Here's how the part is built. I have some questions about the finished solid (model axes, mm). Give positions to 0.01 mm unless a question says otherwise; leave off trailing zeros. Order: outer loops, then holes, each group sorted by start corner. A loop starts at its lowest first (then second) coordinate and runs counter-clockwise, first axis right, second up.
from build123d import *

# Parameters (mm, degrees)
SKETCH1_W           = 73
SKETCH1_H           = 30
SKETCH1_W_2         = 7
SKETCH1_H_2         = 2
SKETCH1_W_3         = 2
SKETCH1_H_3         = 7
BOSS_EXTRUDE1_DEPTH = 2
CUT_EXTRUDE1_DEPTH  = 10
SKETCH6_R           = 2
CUT_EXTRUDE2_DEPTH  = 19


with BuildPart() as part:
    # Sketch1 → Boss-Extrude1 (new body)
    with BuildSketch(Plane(origin=(0, 0, 0), x_dir=(1, 0, 0), z_dir=(0, 1, 0))):
        with Locations((-11.269774173, -9.91409445)):
            Rectangle(SKETCH1_W, SKETCH1_H)
        with Locations((-39.269774173, -16.41409445)):
            Rectangle(SKETCH1_W_2, SKETCH1_H_2, mode=Mode.SUBTRACT)
        with Locations((-39.269774173, -3.41409445)):
            Rectangle(SKETCH1_W_2, SKETCH1_H_2, mode=Mode.SUBTRACT)
        with Locations((16.730225827, -3.41409445)):
            Rectangle(SKETCH1_W_2, SKETCH1_H_2, mode=Mode.SUBTRACT)
        with Locations((16.730225827, -16.41409445)):
            Rectangle(SKETCH1_W_2, SKETCH1_H_2, mode=Mode.SUBTRACT)
        with Locations((-29.769774173, -3.41409445)):
            Rectangle(SKETCH1_W_3, SKETCH1_H_3, mode=Mode.SUBTRACT)
        with Locations((-29.769774173, -16.41409445)):
            Rectangle(SKETCH1_W_3, SKETCH1_H_3, mode=Mode.SUBTRACT)
        with Locations((7.230225827, -16.41409445)):
            Rectangle(SKETCH1_W_3, SKETCH1_H_3, mode=Mode.SUBTRACT)
        with Locations((7.230225827, -3.41409445)):
            Rectangle(SKETCH1_W_3, SKETCH1_H_3, mode=Mode.SUBTRACT)
    extrude(amount=BOSS_EXTRUDE1_DEPTH)

    # Sketch3 → Cut-Extrude1 (cut)
    with BuildSketch(Plane(origin=(0, 2, 0), x_dir=(1, 0, 0), z_dir=(0, 1, 0))):
        Polygon((-20.17963908, -3.41409445), (-22.7291277, -14.91409445), (-17.850525272, -14.91409445), (-12.508752888, -14.91409445), (-7.630150459, -14.91409445), (-10.17963908, -3.41409445), align=None)
        Polygon((-5.138202105, -16.91409445), (-12.508752888, -16.91409445), (-12.508752888, -14.91409445), (-7.630150459, -14.91409445), (-10.17963908, -3.41409445), (-20.17963908, -3.41409445), (-22.7291277, -14.91409445), (-17.850525272, -14.91409445), (-17.850525272, -16.91409445), (-25.221076054, -16.91409445), (-21.784808783, -1.41409445), (-8.574469376, -1.41409445), align=None)
    extrude(amount=-CUT_EXTRUDE1_DEPTH, mode=Mode.SUBTRACT)

    # Sketch6 → Cut-Extrude2 (cut)
    with BuildSketch(Plane(origin=(0, 2, 0), x_dir=(1, 0, 0), z_dir=(0, 1, 0))):
        with Locations(Location((-35.769774173, -9.16409445, 0), (0, 0, 270))):
            Circle(SKETCH6_R)
        with Locations(Location((2.230225827, -9.16409445, 0), (0, 0, 270))):
            Circle(SKETCH6_R)
    extrude(amount=-CUT_EXTRUDE2_DEPTH, mode=Mode.SUBTRACT)


solid = part.part
Q1. Thinking about a two-plate mould opening in X: for faces 1 (the face through (-12, 1, 24.914)), 2 (the face through (6.23, 1, 16)), which applies, released by +X, released by -X, zero draft, split by the parting line, or undercut?
Filled sheet:
face 1: zero draft
face 2: undercut
Q2. I need wall thicknesses on L1, parallel to X at y = 1.5, z = 17.5; L2, parallel to Z at x = -41, y = 1.9; L3, parallel to X at y = 1.75, z = 5. Which ranges of each line are inside material? Lowest first, please.
Filled sheet:
L1: x = -47.77 to -30.77, -28.77 to 6.23, 8.23 to 25.23
L2: z = -5.09 to 2.41, 4.41 to 15.41, 17.41 to 24.91
L3: x = -47.77 to -30.77, -28.77 to -22.58, -7.78 to 6.23, 8.23 to 25.23
Q3. If we section it at C-C on x = -16: List the corners of the cut face in (y, z) for me.
Filled sheet:
outline: (0, -5.09) - (2, -5.09) - (2, 1.41) - (0, 1.41) - close; (0, 14.91) - (2, 14.91) - (2, 24.91) - (0, 24.91) - close
Q4. If we section it at A-A on x = 16: List the corners of the cut face in (y, z) for me.
Filled sheet:
outline: (0, -5.09) - (2, -5.09) - (2, 2.41) - (0, 2.41) - close; (0, 4.41) - (2, 4.41) - (2, 15.41) - (0, 15.41) - close; (0, 17.41) - (2, 17.41) - (2, 24.91) - (0, 24.91) - close
Q5. If we section it at B-B on z = 16.25: List the corners of the cut face in (x, y) for me.
Filled sheet:
outline: (-47.77, 0) - (-42.77, 0) - (-42.77, 2) - (-47.77, 2) - close; (-35.77, 0) - (-30.77, 0) - (-30.77, 2) - (-35.77, 2) - close; (-28.77, 0) - (-25.07, 0) - (-25.07, 2) - (-28.77, 2) - close; (-17.85, 0) - (-12.51, 0) - (-12.51, 2) - (-17.85, 2) - close; (-5.29, 0) - (6.23, 0) - (6.23, 2) - (-5.29, 2) - close; (8.23, 0) - (13.23, 0) - (13.23, 2) - (8.23, 2) - close; (20.23, 0) - (25.23, 0) - (25.23, 2) - (20.23, 2) - close
Q6. If we section it at D-D on z = 9.5: List the corners of the cut face in (x, y) for me, plus the area to 3 significant figures.
Filled sheet:
outline: (-47.77, 0) - (-37.74, 0) - (-37.74, 2) - (-47.77, 2) - close; (-33.8, 0) - (-23.58, 0) - (-23.58, 2) - (-33.8, 2) - close; (-6.78, 0) - (0.26, 0) - (0.26, 2) - (-6.78, 2) - close; (4.2, 0) - (25.23, 0) - (25.23, 2) - (4.2, 2) - close
area: 96.6 mm2
